Part print with two shaded views. Sizes in mm from the minimum x, y, z corner. A direction names the side the tool comes from. Round coordinates to 2 decimals unless told otherwise and drop trailing zeros. Write each loop counter-clockwise with the first axis right and the second up, starting at its lowest first coordinate (ties: lowest second). Pieces come first, ordered by that corner, then holes. Notation, with made-up numbers: (31, 43) -> (36, 43) arc R30 cw to (36, 70) -> close; hole circle Ø4 at (87, 79.25). An arc over 180 degrees is marked (long way). Return JSON: item names as keys, results as strings. Group by question number.
(1) Mould opens along Y. For the marked faces 1, 2 and 3 say: +Y half, -Y half, draft (parallel to the pull), parting line (faces both ways), or undercut.
(2) Saw through at B-B (x = 54.5). List the corners of the cut face in (y, z), plus the area to 3 significant figures.
(3) Drill centre lines: L1, parallel to Y at x = 44.25, z = 10.75; L2, parallel to Y at x = 41, z = 26 (1 decimal); L3, parallel to Z at x = 43.5, y = 31. Where is each one in solid material? Low to high. Write a range as from..to.
(4) Saw through at A-A (z = 18.5). List the corners of the cut face in (x, y) (1 decimal).
(5) Saw through at D-D (z = 10). List the corners of the cut face in (x, y) (1 decimal).
(6) Saw through at C-C (y = 11). List the corners of the cut face in (x, z).
(7) Tool access for the marked faces 4, 5 and 6: list every direction of +Z, -Z, +X, -X, +Y, -Y with a clear straight run to the whole face (end or side of a thin tool).
(8) Drop flat-ended pins along their axis: pin 1 Ø2.5 at (y, z) = (32.5, 26.5) entering from +X; pin 2 Ø1.8 at (y, z) = (31.92, 10.75) entering from +X; pin 3 Ø5 at (x, z) = (7.5, 13) entering from +Y (1 decimal); pin 4 Ø1 at (x, z) = (55, 24.5) entering from +Y. Give the stop position or say it passes through.
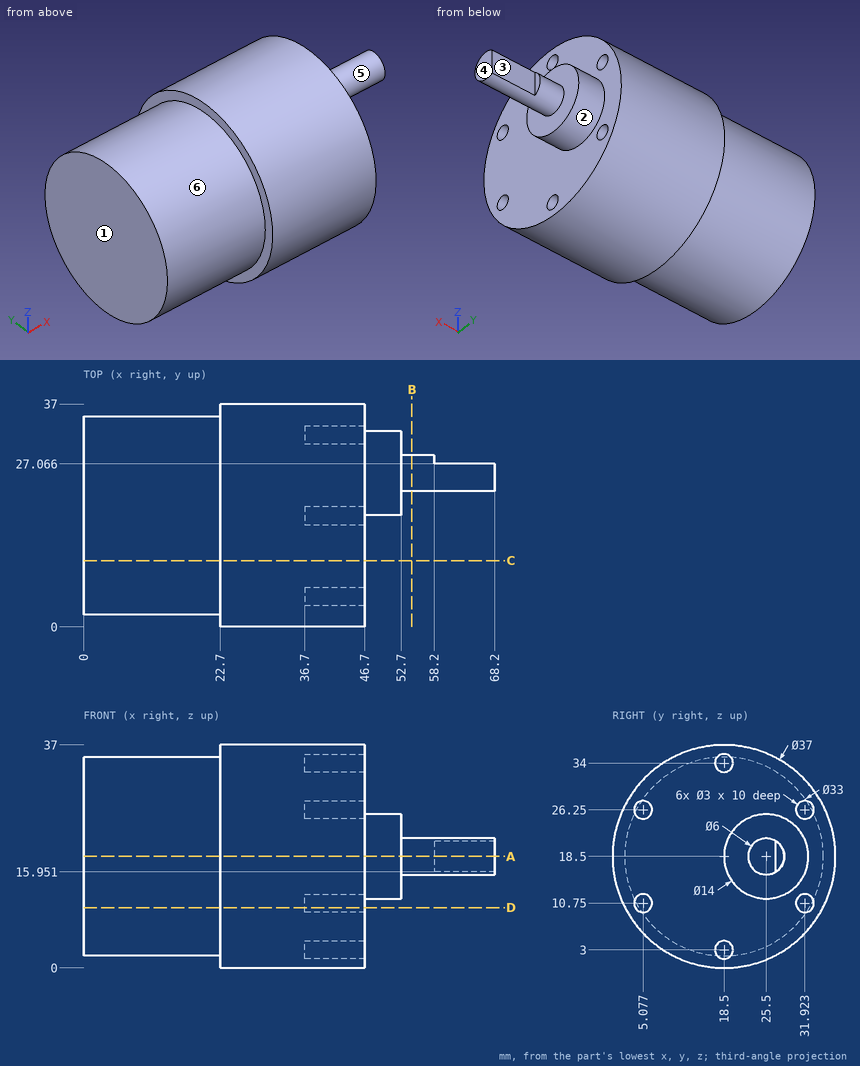
Computed values:
{
 "1": {"face 1": "draft", "face 2": "parting line", "face 3": "+Y half"},
 "2": {"outline": "circle Ø6 at (25.5, 18.5)", "area": "28.3 mm2"},
 "3": {"L1": "1.7..3.58, 6.58..30.42, 33.42..35.3", "L2": "1.6..3.6, 6.6..30.4, 33.4..35.4", "L3": "4.86..9.57, 11.93..25.07, 27.43..32.14"},
 "4": {"outline": "(0, 2) -> (22.7, 2) -> (22.7, 0) -> (46.7, 0) -> (46.7, 18.5) -> (52.7, 18.5) -> (52.7, 22.5) -> (68.2, 22.5) -> (68.2, 27.1) -> (58.2, 27.1) -> (58.2, 28.5) -> (52.7, 28.5) -> (52.7, 32.5) -> (46.7, 32.5) -> (46.7, 37) -> (22.7, 37) -> (22.7, 35) -> (0, 35) -> close"},
 "5": {"outline": "(0, 4.4) -> (22.7, 4.4) -> (22.7, 2.1) -> (46.7, 2.1) -> (46.7, 3.8) -> (36.7, 3.8) -> (36.7, 6.4) -> (46.7, 6.4) -> (46.7, 30.6) -> (36.7, 30.6) -> (36.7, 33.2) -> (46.7, 33.2) -> (46.7, 34.9) -> (22.7, 34.9) -> (22.7, 32.6) -> (0, 32.6) -> close"},
 "6": {"outline": "(0, 3.8) -> (22.7, 3.8) -> (22.7, 1.59) -> (46.7, 1.59) -> (46.7, 35.41) -> (22.7, 35.41) -> (22.7, 33.2) -> (0, 33.2) -> close"},
 "7": {"face 4": "+Z, -Z, +X, +Y, -Y", "face 5": "+X", "face 6": "-X"},
 "8": {"pin 1": "x = 46.7", "pin 2": "x = 36.7", "pin 3": "y = 34.7", "pin 4": "through"}
}
